Source: CAD feature listing. Evaluate the final solid. Frame: model axes, mm. Face numbers are marked on the shaded views. A direction names the side the tool comes from. Give positions to 0.01 mm unless a question says otherwise; leave off trailing zeros. Write each loop counter-clockwise with the first axis right and the second up, starting at its lowest first coordinate (ties: lowest second). Pieces come first, ordered by that corner, then holes. Notation, with made-up numbers: (84.25, 35.5) -> (96.25, 35.5) arc R20 cw to (96.25, 40.5) -> close; hole circle Ø9 at (78, -32). An arc over 180 degrees is marked (long way). Write item = value, one per line.
Autodesk Inventor part; units mm, degrees
ref_plane "YZ Plane" through (0, 0, 0) normal (1, 0, 0) x (0, 1, 0)
ref_plane "XZ Plane" through (0, 0, 0) normal (0, 1, 0) x (-1, 0, 0)
ref_plane "XY Plane" through (0, 0, 0) normal (0, 0, 1) x (1, 0, 0)
sketch "Sketch1" plane through (0, 0, 0) normal (0, 0, 1) x (1, 0, 0)
  line L0 (-22, 20) -> (22, 20)
  line L1 (22, 20) -> (22, 0)
  line L2 (22, 0) -> (-22, 0)
  line L3 (-22, 0) -> (-22, 20)
  line L4 (-22, 20) -> (22, 0) construction
  line L5 (22, 20) -> (-22, 0) construction
  point P0 (0, 0)
  point P1 (0, 10)
  point P2 (0, 10)
  dimension "d0" = 44
  dimension "d1" = 20
extrude "Extrusion1" add sketch "Sketch1" along normal blind 1.5
sketch "Sketch2" plane through (0, 0, 1.5) normal (0, 0, 1) x (1, 0, 0)
  circle A0 centre (-11.5, 10) radius 8
  line L0 (0, -4) -> (0, 24)
  circle A1 centre (11.5, 10) radius 8
  line L1 (-22, 20) -> (-22, 0)
  point P0 (0, 0)
  point P1 (-22, 10)
  point P2 (-19.5, 10)
  dimension "d4" = 16
  dimension "d5" = 2.5
extrude "Extrusion2" add sketch "Sketch2" along normal blind 12.5
sketch "Sketch3" plane through (0, 0, 0) normal (0, 0, -1) x (-1, 0, 0)
  line L0 (21.5, 19.5) -> (-21.5, 19.5)
  line L1 (-21.5, 19.5) -> (-21.5, 0.5)
  line L2 (-21.5, 0.5) -> (21.5, 0.5)
  line L3 (21.5, 0.5) -> (21.5, 19.5)
  line L4 (21.5, 19.5) -> (-21.5, 0.5) construction
  line L5 (-21.5, 19.5) -> (21.5, 0.5) construction
  line L6 (-22, 0) -> (-22, 20)
  line L7 (-22, 20) -> (22, 20)
  line L8 (22, 20) -> (22, 0)
  line L9 (22, 0) -> (-22, 0)
  circle A0 centre (-20.5, 18.5) radius 1
  circle A1 centre (-20.5, 1.5) radius 1
  circle A2 centre (20.5, 18.5) radius 1
  circle A3 centre (20.5, 1.5) radius 1
  point P0 (0, 0)
  point P1 (0, 10)
  dimension "d8" = 0.5
  dimension "d9" = 0.5
  dimension "d10" = 0.5
  dimension "d11" = 0.5
  dimension "d12" = 2
  dimension "d13" = 2
  dimension "d14" = 2
  dimension "d15" = 2
hole "Hole1" at (-20.5, 1.5, 0) at (-20.5, 18.5, 0) at (20.5, 1.5, 0) at (20.5, 18.5, 0) direction (0, 0, 1) diameter 2 depth 6
equation "\"d10\" = d8"
equation "\"d11\" = d9"
equation "\"d13\" = d14"
equation "\"d14\" = d12"
equation "\"d15\" = d12"
equation "\"d16\" = d12"
properties part number "US-015"
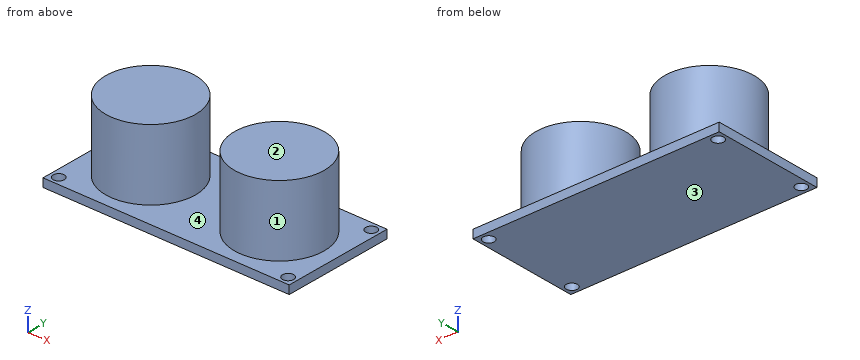
(1) Section query B-B (y = 18.5). Return loops of the section in (x, z).
Values follow:
outline = (-22, 0) -> (-21.5, 0) -> (-21.5, 1.5) -> (-22, 1.5) -> close; (-19.5, 0) -> (19.5, 0) -> (19.5, 1.5) -> (-19.5, 1.5) -> close; (21.5, 0) -> (22, 0) -> (22, 1.5) -> (21.5, 1.5) -> close
(2) Access query for the marked faces 3 and 4. Directions: +Z, -Z, +X, -X, +Y, -Y. A direction counts if a zero-diameter tool reaches every point of the face in a straight line with its end or side. Return the directions, or none.
Values follow:
face_3 = -Z, +X, -X, +Y, -Y
face_4 = +Z
(3) Pull-direction query (X, two-part tool) for the marked faces 1 and 2; classes: pulls with the +X half, pulls with the -X half, needs draft (parallel to the pull), parting line crosses it, or undercut.
Values follow:
face_1 = undercut
face_2 = needs draft
(4) Section query A-A (x = 20.5). Return loops of the section in (y, z), plus the area to 3 significant figures.
Values follow:
outline = (0, 0) -> (0.5, 0) -> (0.5, 1.5) -> (0, 1.5) -> close; (2.5, 0) -> (17.5, 0) -> (17.5, 1.5) -> (2.5, 1.5) -> close; (19.5, 0) -> (20, 0) -> (20, 1.5) -> (19.5, 1.5) -> close
area = 24.0 mm2
(5) Material intervals for line 1 (Y direction, x = 20.5, z = 0.5); line 2 (X direction, y = 1.5, z = 0.7); line 3 (Z direction, x = 17.5, y = 1), sorted ascending.
Values follow:
line_1 = 0 to 0.5, 2.5 to 17.5, 19.5 to 20
line_2 = -22 to -21.5, -19.5 to 19.5, 21.5 to 22
line_3 = 0 to 1.5
(6) Section query D-D (z = 12). Return loops of the section in (x, y).
Values follow:
outline = circle Ø16 at (-11.5, 10); circle Ø16 at (11.5, 10)
(7) First-contact query: pin 1 (2.5 mm diameter, centred on x = 20.5, y = 1.5, fed in from +Z); pin 2 (1.5 mm diameter, centred on y = 17, z = 7, fed in from -X); pin 3 (3 mm diameter, centred on x = 11.5, z = 6, fed in from -Y); pin 4 (1.8 mm diameter, centred on x = 20.5, y = 18.5, fed in from +Z) (1 decimal). Flat tips, straight axial feed; report the tip coordinate or a pass-through.
Values follow:
pin_1 = 1.5
pin_2 = -16.49
pin_3 = 2
pin_4 = through
(8) Section query C-C (y = 10). Return loops of the section in (x, z), plus the area to 3 significant figures.
Values follow:
outline = (-22, 0) -> (22, 0) -> (22, 1.5) -> (19.5, 1.5) -> (19.5, 14) -> (3.5, 14) -> (3.5, 1.5) -> (-3.5, 1.5) -> (-3.5, 14) -> (-19.5, 14) -> (-19.5, 1.5) -> (-22, 1.5) -> close
area = 466 mm2
